from build123d import *

# Parameters (mm, degrees)
SKETCH1_W           = 96
SKETCH1_H           = 52
BOSS_EXTRUDE1_DEPTH = 30
SKETCH3_W           = 30
SKETCH3_H           = 30
CUT_EXTRUDE1_DEPTH  = 10
SKETCH4_W           = 10
SKETCH4_H           = 52
BOSS_EXTRUDE2_DEPTH = 42.5
CUT_EXTRUDE2_DEPTH  = 25
SKETCH6_R           = 1.8
CUT_EXTRUDE3_DEPTH  = 99.250954194
SKETCH7_R           = 10
SKETCH7_R_2         = 4
CUT_EXTRUDE4_DEPTH  = 10
FILLET2_R           = 2
FILLET3_R           = 4
CHAMFER1_SIZE       = 10
CHAMFER1_SIZE2      = 7.002075382
SKETCH10_W          = 6
SKETCH10_H          = 3
CUT_EXTRUDE7_DEPTH  = 124.078227157
SKETCH11_R          = 1.6
SKETCH11_W          = 4
SKETCH11_H          = 32
CUT_EXTRUDE8_DEPTH  = 60


with BuildPart() as part:
    # Sketch1 → Boss-Extrude1 (new body)
    with BuildSketch(Plane(origin=(0, 0, 0), x_dir=(1, 0, 0), z_dir=(0, 1, 0))):
        with Locations((-13, 0)):
            Rectangle(SKETCH1_W, SKETCH1_H)
    extrude(amount=BOSS_EXTRUDE1_DEPTH)

    # Sketch3 → Cut-Extrude1 (cut)
    with BuildSketch(Plane(origin=(0, 30, 0), x_dir=(1, 0, 0), z_dir=(0, 1, 0))):
        with Locations((-2, -2)):
            Rectangle(SKETCH3_W, SKETCH3_H)
    extrude(amount=-CUT_EXTRUDE1_DEPTH, mode=Mode.SUBTRACT)

    # Sketch4 → Boss-Extrude2 (add)
    with BuildSketch(Plane(origin=(0, 30, 0), x_dir=(1, 0, 0), z_dir=(0, 1, 0))):
        with Locations((30, 0)):
            Rectangle(SKETCH4_W, SKETCH4_H)
        with Locations((-56, 0)):
            Rectangle(SKETCH4_W, SKETCH4_H)
    extrude(amount=BOSS_EXTRUDE2_DEPTH)

    # Sketch5 → Cut-Extrude2 (cut)
    with BuildSketch(Plane(origin=(0, 30, 0), x_dir=(1, 0, 0), z_dir=(0, 1, 0))):
        Polygon((25, 22.5), (0.5, 22.5), (0.5, 18), (18, 18), (18, 2.5), (25, 2.5), align=None)
        Polygon((-4.5, 22.5), (-51, 22.5), (-51, 2.5), (-22, 2.5), (-22, 18), (-4.5, 18), align=None)
        Polygon((-22, -2.5), (-51, -2.5), (-51, -22.5), (-22, -22.5), (-22, -20), align=None)
        Polygon((25, -22.5), (25, -2.5), (18, -2.5), (18, -20), (18, -22.5), align=None)
    extrude(amount=-CUT_EXTRUDE2_DEPTH, mode=Mode.SUBTRACT)

    # Sketch6 → Cut-Extrude3 (cut, through all)
    with BuildSketch(Plane.XZ):
        with Locations(Location((-2, 0, 0), (0, 0, 270))):
            Circle(SKETCH6_R)
    extrude(amount=-CUT_EXTRUDE3_DEPTH, mode=Mode.SUBTRACT)

    # Sketch7 → Cut-Extrude4 (cut)
    with BuildSketch(Plane.XZ):
        with Locations(Location((-2, 0, 0), (0, 0, 270))):
            Circle(SKETCH7_R)
        with Locations(Location((-2, 0, 0), (0, 0, 270))):
            Circle(SKETCH7_R_2, mode=Mode.SUBTRACT)
    extrude(amount=-CUT_EXTRUDE4_DEPTH, mode=Mode.SUBTRACT)

    # Fillet2
    fillet2_edges = [part.edges().sort_by_distance(p)[0] for p in [
        (-2, 10, 4),
    ]]
    fillet(fillet2_edges, radius=FILLET2_R)

    # Fillet3
    fillet3_edges = [part.edges().sort_by_distance(p)[0] for p in [
        (-2, 10, 10),
    ]]
    fillet(fillet3_edges, radius=FILLET3_R - 0.0001)  # a hair under: the kernel refuses the full size

    # Chamfer1
    chamfer1_edges = [part.edges().sort_by_distance(p)[0] for p in [
        (-2, 20, 1.8),
    ]]
    chamfer1_side = [part.faces().sort_by_distance(p)[0] for p in [
        (-2, 20, 2.022878214),
    ]]
    chamfer(chamfer1_edges, length=CHAMFER1_SIZE, length2=CHAMFER1_SIZE2, reference=chamfer1_side[0])

    # Sketch10 → Cut-Extrude7 (cut, through all)
    with BuildSketch(Plane(origin=(35, 0, 0), x_dir=(0, 0, -1), z_dir=(1, 0, 0))):
        with Locations((21, 61)):
            Rectangle(SKETCH10_W, SKETCH10_H)
        with Locations((-21, 61)):
            Rectangle(SKETCH10_W, SKETCH10_H)
    extrude(amount=-CUT_EXTRUDE7_DEPTH, mode=Mode.SUBTRACT)

    # Sketch11 → Cut-Extrude8 (cut)
    with BuildSketch(Plane(origin=(0, 72.5, 0), x_dir=(1, 0, 0), z_dir=(0, 1, 0))):
        with Locations(Location((-56, 21, 0), (0, 0, 270))):
            Circle(SKETCH11_R)
        with Locations(Location((-56, -21, 0), (0, 0, 270))):
            Circle(SKETCH11_R)
        with Locations(Location((30, -21, 0), (0, 0, 270))):
            Circle(SKETCH11_R)
        with Locations(Location((30, 21, 0), (0, 0, 270))):
            Circle(SKETCH11_R)
        with Locations((-56, 0)):
            Rectangle(SKETCH11_W, SKETCH11_H)
        with Locations((30, 0)):
            Rectangle(SKETCH11_W, SKETCH11_H)
    extrude(amount=-CUT_EXTRUDE8_DEPTH, mode=Mode.SUBTRACT)


solid = part.part
Geometry: final body of the model. Coordinates: model frame, mm. A direction names the side the tool comes from. Give positions to 0.01 mm unless a question says otherwise; leave off trailing zeros. Loops run counter-clockwise (first coordinate to the right, second up) from the corner with the lowest first, then second, coordinate; pieces in that order, holes last. Notation, with made-up numbers: (-17, 52) -> (-8, 52) arc R33 ccw to (-8, 87) -> close; hole circle Ø7 at (16.25, -11). An arc over 180 degrees is marked (long way). Put each result on its own line as item: value.
1. Cut plane A-A (y = 43.5). Return the cut outline in (x, z), plus the area to 3 significant figures.
Taken from the geometry:
outline: (-61, -26) -> (-51, -26) -> (-51, 26) -> (-61, 26) -> close; (25, -26) -> (35, -26) -> (35, 26) -> (25, 26) -> close; hole (-58, -16) -> (-54, -16) -> (-54, 16) -> (-58, 16) -> close; hole circle Ø3.2 at (-56, -21); hole circle Ø3.2 at (-56, 21); hole (28, -16) -> (32, -16) -> (32, 16) -> (28, 16) -> close; hole circle Ø3.2 at (30, -21); hole circle Ø3.2 at (30, 21)
area: 752 mm2
2. Set-up query: faces 5 (the cylindrical face through (1.966, 3.944, 0.521)), 6 (the flat face through (28, 43, 0)), 7 (the flat face through (-54.8, 59.5, 19.7)). Return all of +Z, -Z, +X, -X, +Y, -Y with unobstructed straight access to the full face (end or side cutting, diameter ignored); none if empty.
Taken from the geometry:
face 5: -Y
face 6: +Y
face 7: +X, -X
3. Ray query, line 1 along X through (y, z) = (46, -21); line 2 along X through (y, z) = (37.5, 12); line 3 along Z through (x, y) = (20.5, 13). Return the intervals inside material, ascending. Write a range as [from, to].
Taken from the geometry:
line 1: x = [-61, -57.6], [-54.4, -51], [25, 28.4], [31.6, 35]
line 2: x = [-61, -58], [-54, -51], [25, 28], [32, 35]
line 3: z = [-26, -22.5], [-2.5, 2.5], [22.5, 26]
4. Pin query (flat end, axial travel): P1, Ø3, axis at x = -57, z = -3.5, coming from the +Y side; P2, Ø1, axis at x = -34, z = 13.5, coming from the +Y side; P3, Ø3, axis at x = -56, z = -21, coming from the +Y side. Return the tip coordinate at first contact, or that it passes through.
Taken from the geometry:
P1: stops at y = 72.5
P2: stops at y = 5
P3: stops at y = 12.5
5. Pull-direction query (Y, two-part tool) for faces 1 (the flat face through (-14, 0, 0)), 2 (the flat face through (-54.8, 62.5, 19.7)), 3 (the flat face through (25, 38, 0)), 4 (the flat face through (-33, 5, -13)); classes: released by +Y, released by -Y, zero draft, split by the parting line, or undercut.
Taken from the geometry:
face 1: released by -Y
face 2: undercut
face 3: zero draft
face 4: released by +Y
6. Cut plane D-D (x = -33.5). Return the cut outline in (y, z).
Taken from the geometry:
outline: (0, -26) -> (30, -26) -> (30, -22.5) -> (5, -22.5) -> (5, -2.5) -> (30, -2.5) -> (30, 2.5) -> (5, 2.5) -> (5, 22.5) -> (30, 22.5) -> (30, 26) -> (0, 26) -> close
7. Cut plane B-B (x = 11). Return the cut outline in (y, z), plus the area to 3 significant figures.
Taken from the geometry:
outline: (0, -26) -> (30, -26) -> (30, -22.5) -> (5, -22.5) -> (5, -18) -> (30, -18) -> (30, -13) -> (20, -13) -> (20, 17) -> (30, 17) -> (30, 26) -> (0, 26) -> close
area: 1,150 mm2
8. Cut plane C-C (z = 21). Count the separate pieces of the cut face and the enclosed holes in it, plus the area to 3 significant figures.
Taken from the geometry:
separate pieces: 5
enclosed holes: 0
area: 2,410 mm2
